Work out the finished part from the listing and answer in its coordinate system (mm). A direction names the side the tool comes from. Give positions to 0.01 mm unless a question says otherwise; leave off trailing zeros. Loops run counter-clockwise (first coordinate to the right, second up) from the corner with the lowest first, then second, coordinate; pieces in that order, holes last. Notation, with made-up numbers: M 30,31 L 48,31 A14 ccw 48,44 Z; hole C 25.25,-33.5 d3. An arc over 180 degrees is marked long. Write item = value, one per line. Start each with the question number.
1. For faces 1 (the face through (11.923, -2.493, -3.755)), 2 (the face through (-5, 0, -9)), determine the directions among +Z, -Z, +X, -X, +Y, -Y from which every point of the face is accessible in a straight line to the end or side of a thin tool.
2. Flat-ended cylindrical pins translate along their axes: pin 1 Ø12 at (x, y) = (-6.5, 18) entering from -Z; pin 2 Ø1 at (y, z) = (46.5, -3.5) entering from -X; pin 3 Ø5 at (x, y) = (3.5, 37) entering from -Z. Find the tip coordinate at first contact, or state that the pin passes through.
3. Consider L1, parallel to Y at x = 9.5, z = -2.25; L2, parallel to Y at x = 0, z = -11; L3, parallel to Z at x = 6.25, y = 0.5. Determine where each line is inside the solid, lowest interval first. Write a range as [from, to].
4. Section B-B on y = 2.5 is taken. Determine the outline of the cut face in (x, z).
5. Section A-A on x = 0 is taken. Determine the outline of the cut face in (y, z).
Autodesk Inventor part; units mm, degrees
ref_plane "YZ Plane" through (0, 0, 0) normal (1, 0, 0) x (0, 1, 0)
ref_plane "XZ Plane" through (0, 0, 0) normal (0, 1, 0) x (-1, 0, 0)
ref_plane "XY Plane" through (0, 0, 0) normal (0, 0, 1) x (1, 0, 0)
sketch "Sketch1" plane through (0, 0, 0) normal (0, 1, 0) x (-1, 0, 0)
  circle A0 centre (0, 0) radius 9.5
  dimension "d0" = 19
extrude "Extrusion1" add sketch "Sketch1" along normal blind 55
sketch "Sketch2" plane through (0, 0, 0) normal (0, -1, 0) x (1, 0, 0)
  point P0 (0, 0)
sketch "Sketch3" plane through (0, 0, 0) normal (0, -1, 0) x (1, 0, 0)
  circle A0 centre (0, 0) radius 12.5
  dimension "d3" = 25
extrude "Extrusion2" add sketch "Sketch3" along normal blind 5
fillet "Fillet1" radius 2 2 edges at (-12.5, 0, 0) (-12.5, -5, 0)
sketch "Sketch4" plane through (0, 55, 0) normal (0, 1, 0) x (1, 0, 0)
  point P0 (0, 0)
sketch "Sketch5" plane through (0, 0, 0) normal (0, 1, 0) x (1, 0, 0)
  point P0 (0, 0)
sketch "Sketch6" plane through (0, 0, 0) normal (1, 0, 0) x (0, 1, 0)
  point P0 (0, 0)
equation "\"BendRadius\" = Thickness"
equation "\"BendReliefWidth\" = Thickness"
equation "\"BendReliefDepth\" = 0.5 * Thickness"
equation "\"CornerReliefSize\" = 4 * Thickness"
equation "\"MinimumRemnant\" = 2 * Thickness"
equation "\"TransitionRadius\" = BendRadius"
equation "\"JacobiRadiusSize\" = BendRadius"
equation "\"GapSize\" = Thickness"
Verdict:
q1.face_1 = +Y, -Y
q1.face_2 = +Y
q2.pin_1 = -9.49
q2.pin_2 = -9.01
q2.pin_3 = -9.45
q3.L1 = [-5, 0]
q3.L2 = [-4.94, -0.06]
q3.L3 = [-7.15, 7.15]
q4.outline = C 0,0 d19
q5.outline = M -5,-10.5 A2 ccw -3,-12.5 L -2,-12.5 A2 ccw 0,-10.5 L 0,-9.5 L 55,-9.5 L 55,9.5 L 0,9.5 L 0,10.5 A2 ccw -2,12.5 L -3,12.5 A2 ccw -5,10.5 Z
